Work out the finished part from the listing and answer in its coordinate system (mm). A direction names the side the tool comes from. Round coordinates to 2 decimals unless told otherwise and drop trailing zeros. Write each loop counter-clockwise with the first axis right and the second up, starting at its lowest first coordinate (ties: lowest second). Pieces come first, ordered by that corner, then holes.
1. A tool of negligible diameter and unlimited length cuts with its end or side. For faces 1 (the face through (7.3, 7.3, 98.9)), 2 (the face through (-9.76, -2.17, -48.76)), 3 (the face through (0.755, -19.225, 62.06)), from which of +Z, -Z, +X, -X, +Y, -Y can it reach the whole face along a straight path? Write none if from no direction.
2. Find section A-A (z = 96). Write down the section's boundary in (x, y), and give its area (3 significant figures).
3. Find section C-C (z = 132.5). Write down the section's boundary in (x, y).
4. Straight lines are drawn through the part: probe 1 along X at (y, z) = (0, 144.25); probe 2 along Y at (x, z) = (0, 148); probe 3 along Z at (x, y) = (-4, 20). For each, find the intervals that lie inside material, in ascending order.
5. Flat-ended cylindrical pins translate along their axes: pin 1 Ø14 at (x, z) = (-3.5, 67) entering from +Y; pin 2 Ø1 at (x, z) = (-2.5, 82) entering from +Y; pin 3 Ø0.6 at (x, y) = (1.5, 8.5) entering from +Z; pin 4 Ø10 at (x, y) = (2.5, -2) entering from +Z. Find the tip coordinate at first contact, or state that the pin passes through.
6. Find section B-B (z = -5). Write down the section's boundary in (x, y).
7. Determine the mould class of faces 4 (the face through (0.753, -19.986, 69.54)), 5 (the face through (4, 9, -46.7)), 6 (the face through (0.342, -9.167, 154.626)) for opening direction Z: pulls with the +Z half, pulls with the -Z half, needs draft (parallel to the pull), parting line crosses it, or undercut.
Autodesk Inventor part; units mm, degrees
ref_plane "Wellennuttiefe_Arbeitsebene_2" through (0, 6.5, 126.35) normal (0, 1, 0) x (-1, 0, 0)
ref_plane "YZ Plane" through (0, 0, 0) normal (1, 0, 0) x (0, 1, 0)
ref_plane "XY Plane" through (0, 0, 0) normal (0, 0, 1) x (1, 0, 0)
sketch "Skizze1" plane through (0, 0, 0) normal (1, 0, 0) x (0, 1, 0)
  line L0 (0, 154.8) -> (9, 154.8)
  line L1 (9, 154.8) -> (10, 153.8)
  line L2 (10, 153.8) -> (10, 98.9)
  line L3 (18, 75.9) -> (20, 73.9)
  line L4 (20, 73.9) -> (20, 65.3)
  line L5 (20, 61.3) -> (20, 41.1)
  line L6 (20, 41.1) -> (23.5, 41.1)
  line L7 (23.5, 41.1) -> (23.5, 36.1)
  line L8 (23.5, 36.1) -> (16.5, 36.1)
  line L9 (16.5, 36.1) -> (16.5, -13.8)
  line L10 (10, -15.8) -> (10, -46.7)
  line L11 (10, -46.7) -> (9.5, -46.7)
  line L12 (9.5, -46.7) -> (9.5, -48)
  line L13 (9.5, -48) -> (10, -48)
  line L14 (10, -48) -> (10, -49.5)
  line L15 (10, -49.5) -> (9.5, -50)
  line L16 (9.5, -50) -> (0, -50)
  line L17 (0, -50) -> (0, 154.8)
  line L18 (14.5, -15.8) -> (10, -15.8)
  line L19 (16.5, -13.8) -> (14.5, -15.8)
  line L20 (0, 195.76) -> (0, -90.96) construction
  line L21 (-4.7, 0) -> (28.2, 0) construction
  line L22 (10, 98.9) -> (0, 98.9) construction
  line L23 (10, -15.8) -> (0, -15.8) construction
  line L24 (10, -46.7) -> (0, -46.7) construction
  line L25 (17, 98.9) -> (10, 98.9)
  line L26 (18, 75.9) -> (18, 97.9)
  line L27 (18, 97.9) -> (17, 98.9)
  line L28 (10, 129.8) -> (0, 129.8) construction
  circle A0 centre (20, 63.3) radius 2 construction
  line L29 (20, 65.3) -> (19.0799, 64.3799)
  line L30 (19.0799, 64.3799) -> (19.0799, 62.2201)
  line L31 (19.0799, 62.2201) -> (20, 61.3)
  line L32 (20, 63.3) -> (19.0799, 63.3) construction
  line L33 (18, 75.9) -> (18, 75.9)
  point P0 (0, 0)
  point P1 (18, 98.9)
  dimension "d4" = 45
  dimension "d6" = 1.3
  dimension "d9" = 23.5
  dimension "d11" = 5
  dimension "d19" = 45
  dimension "d21" = 2
  dimension "d22" = 1
  dimension "d34" = 0
  dimension "d35" = 50
  dimension "d36" = 45
  dimension "d87" = 114.7
  dimension "d88" = 0
  dimension "d89" = 30.9
  dimension "d90" = 19
  dimension "d91" = 20
  dimension "d119" = 20
  dimension "d120" = 1.5
  dimension "d122" = 1
  dimension "d123" = 1
  dimension "d124" = 33
  dimension "d125" = 40
  dimension "d126" = 30.9
  dimension "d127" = 25
  dimension "d135" = 78.9
  dimension "d139" = 91.5
  dimension "d140" = 113.7
  dimension "d141" = 22.2
  dimension "d142" = 45
  dimension "d143" = 45
  dimension "d144" = 38.1598
  dimension "d145" = 8.6
  dimension "d157" = 36
  dimension "d158" = 2
revolve "Umdrehung1" add sketch "Skizze1" angle 360 about axis through (0, 0, -50) along (0, 0, 1)
ref_plane "Wellennuttiefe_Arbeitsebene" through (0, 15, 51.2) normal (0, 1, 0) x (-1, 0, 0)
ref_plane "Arbeitsebene1" through (0, 20, 51.2) normal (0, 1, 0) x (-1, 0, 0)
sketch "Skizze2" plane through (0, 20, 51.2) normal (0, 1, 0) x (-1, 0, 0)
  line L0 (-23.5, -10.1) -> (23.5, -10.1) construction
  line L1 (0, 144.56) -> (0, -142.16) construction
  line L2 (20, 10.1) -> (20, -10.1) construction
  line L3 (-20, 10.1) -> (-20, -10.1) construction
  line L4 (-19.0799, 11.0201) -> (19.0799, 11.0201) construction
  line L5 (20, -10.1) -> (-20, -10.1)
  line L6 (-20, -10.1) -> (-20, 47.7)
  line L7 (-20, 47.7) -> (20, 47.7)
  line L8 (20, 47.7) -> (20, -10.1)
  line L9 (-16.5, 24.7) -> (16.5, 24.7) construction
  line L10 (-17, 47.7) -> (17, 47.7) construction
  point P0 (0, -51.2)
extrude "Passfeder_Ausnahme" cut sketch "Skizze2" against normal blind 2
thread "Gewinde1"
ref_plane "Arbeitsebene5" through (0, 10, 126.35) normal (0, 1, 0) x (-1, 0, 0)
sketch "Skizze7" plane through (0, 10, 126.35) normal (0, 1, 0) x (-1, 0, 0)
  line L0 (-10, -27.45) -> (10, -27.45) construction
  line L1 (10, 3.45) -> (-10, 3.45) construction
  line L2 (-10, -27.45) -> (10, -27.45) construction
  line L3 (0, -27.45) -> (0, 3.45) construction
  line L4 (10, 27.45) -> (10, -27.45) construction
  line L5 (-10, 27.45) -> (-10, -27.45) construction
  line L6 (-9, 28.45) -> (9, 28.45) construction
  line L7 (-17, -27.45) -> (17, -27.45) construction
  line L8 (0, 28.45) -> (0, 3.45) construction
  line L9 (10, 3.45) -> (-10, 3.45)
  line L10 (-10, 3.45) -> (-10, 28.45)
  line L11 (-10, 28.45) -> (10, 28.45)
  line L12 (10, 28.45) -> (10, 3.45)
  point P0 (0, -126.35)
  dimension "d100" = 30.9
  dimension "Flansch_Max_Connector_Lenght" = 25
ref_plane "Wellennuttiefe_Arbeitsebene_2" through (0, 6.5, 126.35) normal (0, 1, 0) x (-1, 0, 0)
extrude "Flachstelle_Flansch" cut sketch "Skizze7" against normal blind 2
sketch "Skizze9" plane through (0, 0, 154.8) normal (0, 0, 1) x (1, 0, 0)
  circle A0 centre (0, 0) radius 9 construction
  point P0 (0, 0)
hole "Bohrung1" at (0, 0, 154.8) direction (0, 0, -1) diameter 4.134 depth 15 tip angle 118
chamfer "Fase4" distance 1.5 angle 45 1 edges at (0, 2.067, 154.8)
sketch "Skizze11" plane through (-25.5, 0, 153.8) normal (0, 0, 1) x (1, 0, 0)
  arc A0 (0, 0) -> (51, 0) centre (25.5, 0) ccw
  circle A1 centre (25.5, 0) radius 23.5
  line L0 (0, -25.5) -> (51, -25.5)
  line L1 (51, -25.5) -> (51, 0)
  line L2 (0, -25.5) -> (0, 0)
  point P0 (25.5, 0)
  point P1 (25.5, -25.5)
sketch "Skizze12" plane through (0, 0, 153.8) normal (0, 0, 1) x (1, 0, 0)
  circle A0 centre (0, 0) radius 16.5
  circle A1 centre (0, 0) radius 16.5
  line L0 (-25.5, -25.5) -> (25.5, -25.5)
  line L1 (-10, 0) -> (-25.5, 0)
  line L2 (-25.5, 0) -> (-25.5, -25.5)
  line L3 (-25.5, -25.5) -> (25.5, -25.5)
  line L4 (25.5, -25.5) -> (25.5, 0)
  line L5 (10, 0) -> (25.5, 0)
  arc A2 (-10, 0) -> (10, 0) centre (0, 0) ccw
  circle A3 centre (0, 0) radius 15.7
  line L6 (-17, 0) -> (-10, 0)
  line L7 (-15.7, 0) -> (-15.7, -25.5)
  line L8 (-25.5, -25.5) -> (25.5, -25.5)
  line L9 (10, 0) -> (25.5, 0)
  line L10 (15.7, 0) -> (15.7, -25.5)
  point P0 (0, 0)
  point P1 (25.5, -25.5)
  point P2 (15.7, 0)
  point P3 (-15.7, 0)
  dimension "d155" = 0.8
sketch "Skizze10" plane through (0, 0, 0) normal (1, 0, 0) x (0, 1, 0)
  line L0 (-18, 75.9) -> (-18, 97.9)
  line L1 (-18, 97.9) -> (-17, 98.9)
  line L2 (-17, 98.9) -> (-10, 98.9)
  line L3 (-10, 98.9) -> (-10, 153.8)
  line L4 (-10, 153.8) -> (-9, 154.8)
  line L5 (-9, 154.8) -> (-3.567, 154.8)
  line L6 (-3.567, 154.8) -> (-2.067, 153.3)
  line L7 (-2.067, 153.3) -> (-2.067, 139.8)
  line L8 (-2.067, 139.8) -> (0, 138.558)
  line L9 (0, 138.558) -> (2.067, 139.8)
  line L10 (2.067, 139.8) -> (2.067, 153.3)
  line L11 (2.067, 153.3) -> (3.567, 154.8)
  line L12 (3.567, 154.8) -> (6.5, 154.8)
  line L13 (6.5, 154.8) -> (6.5, 129.8)
  line L14 (6.5, 129.8) -> (10, 129.8)
  line L15 (10, 129.8) -> (10, 98.9)
  line L16 (10, 98.9) -> (17, 98.9)
  line L17 (17, 98.9) -> (18, 97.9)
  line L18 (18, 97.9) -> (18, 75.9)
  line L19 (18, 75.9) -> (20, 73.9)
  line L20 (20, 73.9) -> (20, 65.3)
  line L21 (20, 65.3) -> (19.0799, 64.3799)
  line L22 (19.0799, 64.3799) -> (19.0799, 62.2201)
  line L23 (19.0799, 62.2201) -> (15, 62.2201)
  line L24 (15, 62.2201) -> (15, 41.1)
  line L25 (15, 41.1) -> (23.5, 41.1)
  line L26 (23.5, 41.1) -> (23.5, 36.1)
  line L27 (23.5, 36.1) -> (16.5, 36.1)
  line L28 (16.5, 36.1) -> (16.5, -13.8)
  line L29 (16.5, -13.8) -> (14.5, -15.8)
  line L30 (14.5, -15.8) -> (10, -15.8)
  line L31 (10, -15.8) -> (10, -46.7)
  line L32 (10, -46.7) -> (9.5, -46.7)
  line L33 (9.5, -46.7) -> (9.5, -48)
  line L34 (9.5, -48) -> (10, -48)
  line L35 (10, -48) -> (10, -49.5)
  line L36 (10, -49.5) -> (9.5, -50)
  line L37 (9.5, -50) -> (-9.5, -50)
  line L38 (-9.5, -50) -> (-10, -49.5)
  line L39 (-10, -49.5) -> (-10, -48)
  line L40 (-10, -48) -> (-9.5, -48)
  line L41 (-9.5, -48) -> (-9.5, -46.7)
  line L42 (-9.5, -46.7) -> (-10, -46.7)
  line L43 (-10, -46.7) -> (-10, -15.8)
  line L44 (-10, -15.8) -> (-14.5, -15.8)
  line L45 (-14.5, -15.8) -> (-16.5, -13.8)
  line L46 (-16.5, -13.8) -> (-16.5, 36.1)
  line L47 (-16.5, 36.1) -> (-23.5, 36.1)
  line L48 (-23.5, 36.1) -> (-23.5, 41.1)
  line L49 (-23.5, 41.1) -> (-20, 41.1)
  line L50 (-20, 41.1) -> (-20, 61.3)
  line L51 (-20, 61.3) -> (-19.0799, 62.2201)
  line L52 (-19.0799, 62.2201) -> (-19.0799, 64.3799)
  line L53 (-19.0799, 64.3799) -> (-20, 65.3)
  line L54 (-20, 65.3) -> (-20, 73.9)
  line L55 (-20, 73.9) -> (-18, 75.9)
  line L56 (-10, 153.8) -> (6.5, 153.8)
  line L57 (-10, 153.8) -> (-25.5, 153.8)
  line L58 (-25.5, 153.8) -> (-25.5, -13.8)
  line L59 (-16.5, 36.1) -> (-16.5, -13.8)
  line L60 (0, -90.96) -> (0, 195.76)
  line L61 (-20, 61.3) -> (-20, 41.1)
  line L62 (-25.5, -13.8) -> (-16.5, -13.8)
  point P0 (0, 0)
  point P1 (2.567, 153.8)
  point P2 (-2.567, 153.8)
  dimension "d154" = 2
equation "\"d100\" = MainAxis_Bearing_Fix2ScrewLimit_Dist + MainAxis_Bearing_Fix2Limit_Dist"
equation "\"d6\" = Sprengring_NutBreite"
equation "\"d87\" = -MainAxis_Bearing_Fix2ScrewLimit_Dist + Gestell_Lager_Distanz - MainAxis_Bearing_Fix2Limit_Dist"
equation "\"d89\" = MainAxis_Bearing_Fix2Limit_Dist + MainAxis_Bearing_Fix2ScrewLimit_Dist"
equation "\"d90\" = Sprengring_NutDurchmesser"
equation "\"d91\" = P204_ShaftDiameter"
equation "\"d119\" = P204_ShaftDiameter"
equation "\"Wellennuttiefe_20\" = 3.5"
equation "\"Nabennuttiefe_20\" = 2.8"
equation "\"Sprengring_NutBreite\" = 1.3"
equation "\"Sprengring_NutDurchmesser\" = 19"
equation "\"Nabennuttiefe_40\" = 3.3"
equation "\"Wellennuttiefe_40\" = 5"
equation "\"Passfeder_Width_20\" = 6"
equation "\"Passfeder_Width_40\" = 12"
properties part number "Welle_Flachstelle" material "Edelstahl"
Worked answers:
1. face 1: +Z
1. face 2: -Z
1. face 3: none
2. outline: circle Ø36 at (0, 0)
2. area: 1,020 mm2
3. outline: (-6, 8) arc R10 ccw (long way) to (6, 8) - close
4. probe 1: x = -10 to -2.07, 2.07 to 10
4. probe 2: y = -10 to -2.07, 2.07 to 8
4. probe 3: z = 36.1 to 41.1
5. pin 1: stops at y = 18
5. pin 2: stops at y = 17.89
5. pin 3: stops at z = 129.8
5. pin 4: stops at z = 154.8
6. outline: circle Ø33 at (0, 0)
7. face 4: needs draft
7. face 5: undercut
7. face 6: pulls with the +Z half
